Input: part model. Units: mm. Frame: model coordinates. Face numbers are marked on the shaded views. A direction names the side the tool comes from. Coordinates: 2 decimals unless noted, no trailing zeros. Write each loop counter-clockwise with the first axis right and the second up, starting at its lowest first coordinate (ties: lowest second). Pieces come first, ordered by that corner, then holes. Notation, with made-up numbers: M 87.25,-18.75 L 142.25,-18.75 A12 ccw 142.25,-11.75 Z; hole C 28.25,36.5 d3. An arc over 180 degrees is marked long. Use one line per item in the form item = value.
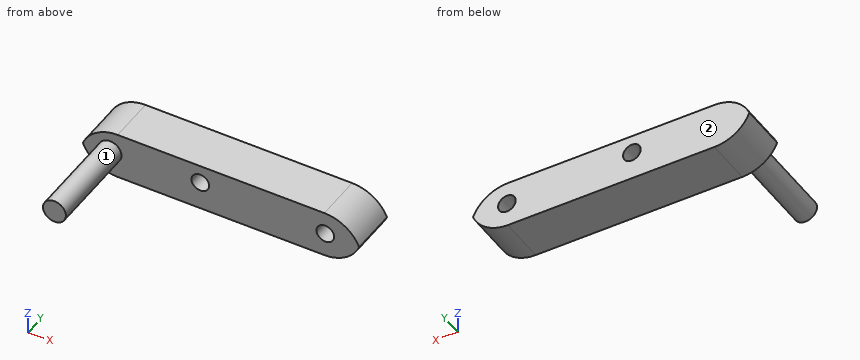
from build123d import *

# Parameters (mm, degrees)
F0_W        = 38.1
F0_H        = 6.35
F0_R        = 1.1938
F1_DEPTH    = 6.35
F2_T1_DEPTH = 31.75
F3_R        = 1.547841459
F4_DEPTH    = 12.7


# Not quite as in the source:
# - a fillet or chamfer that OpenCascade refuses, or shapes differently, is made with other operations: its cross-section is extruded or revolved along the edge and cut away or added


with BuildPart() as f1:
    # F0 (on Front) → F1 (new body)
    with BuildSketch(Plane.XZ):
        with Locations((19.05, 3.175)):
            Rectangle(F0_W, F0_H)
        with Locations((16.2474811077, 3.8697349373)):
            Circle(F0_R, mode=Mode.SUBTRACT)
        with Locations((33.1476069987, 3.302)):
            Circle(F0_R, mode=Mode.SUBTRACT)
    extrude(amount=F1_DEPTH)

    # F2: fillet of radius 5.08 on 4 edges, made by hand

    # F2_s2 → F2_t1 (cut)
    with BuildSketch(Plane.XZ.offset(-12.7)):
        with BuildLine():
            ThreePointArc((0, 1.27), (1.4878975516, 4.8621024484), (5.08, 6.35))
            Line((5.08, 6.35), (0, 6.35))
            Line((0, 6.35), (0, 1.27))
        make_face()
        with BuildLine():
            ThreePointArc((0, 5.08), (1.4878975516, 1.4878975516), (5.08, 0))
            Line((5.08, 0), (0, 0))
            Line((0, 0), (0, 5.08))
        make_face()
        with BuildLine():
            ThreePointArc((38.1, 1.27), (36.6121024484, 4.8621024484), (33.02, 6.35))
            Line((33.02, 6.35), (38.1, 6.35))
            Line((38.1, 6.35), (38.1, 1.27))
        make_face()
        with BuildLine():
            ThreePointArc((33.02, 0), (36.6121024484, 1.4878975516), (38.1, 5.08))
            Line((38.1, 5.08), (38.1, 0))
            Line((38.1, 0), (33.02, 0))
        make_face()
    extrude(amount=F2_T1_DEPTH, mode=Mode.SUBTRACT)

    # F3 (on face) → F4 (join)
    with BuildSketch(Plane.XZ.offset(6.35)):
        with Locations((4.0558986366, 3.4221061505)):
            Circle(F3_R)
    extrude(amount=F4_DEPTH)


solid = f1.part
(1) Section query C-C on x = 21.5. Return the cut outline in (y, z).
Computed:
outline = M -6.35,0 L 0,0 L 0,6.35 L -6.35,6.35 Z
(2) Section query A-A on x = 34. Return the cut outline in (y, z), plus the area to 3 significant figures.
Computed:
outline = M -6.35,0.1 L 0,0.1 L 0,2.47 L -6.35,2.47 Z; M -6.35,4.14 L 0,4.14 L 0,6.25 L -6.35,6.25 Z
area = 28.5 mm^2
(3) Line query: probe 1 along X at (y, z) = (-6, 4); probe 2 along Y at (x, z) = (14, 4). Output: solid intervals per line, ascending.
Computed:
probe_1 = 0.8 to 15.06, 17.43 to 32.18, 34.12 to 37.3
probe_2 = -6.35 to 0
(4) Section query D-D on z = 1. Return the cut outline in (x, y), plus the area to 3 significant figures.
Computed:
outline = M 2.05,-6.35 L 36.05,-6.35 L 36.05,0 L 2.05,0 Z
area = 216 mm^2
(5) First-contact query: pin 1 Ø8 at (x, y) = (21, -13.5) entering from -Z; pin 2 Ø1 at (x, z) = (19.5, 4.5) entering from -Y. Flat tips, straight axial feed; report the tip coordinate or a pass-through.
Computed:
pin_1 = through
pin_2 = -6.35
(6) Section query B-B on y = -2. Return the cut outline in (x, z) (3 decimals).
Computed:
outline = M 0.371,3.175 A5.08 ccw 5.08,0 L 33.02,0 A5.08 ccw 37.729,3.175 A5.08 ccw 33.02,6.35 L 5.08,6.35 A5.08 ccw Z; hole C 16.247,3.87 d2.388; hole C 33.148,3.302 d2.388
(7) Set-up query: the marked faces 1 and 2. Return all of +Z, -Z, +X, -X, +Y, -Y with unobstructed straight access to the full face (end or side cutting, diameter ignored); none if empty.
Computed:
face_1 = -Y
face_2 = +Z, -Z, +X, -X, +Y
